```python
from build123d import *

# Parameters (mm, degrees)
SKETCH1_R           = 12.954
SKETCH1_R_2         = 2.25
SKETCH1_R_3         = 14.2748
SKETCH1_R_4         = 1.8415
BOSS_EXTRUDE1_DEPTH = 3.175
FILLET1_R           = 22.479
FILLET2_START       = -1
FILLET2_DEPTH       = 5
FILLET2_2_DEPTH     = 3.175


with BuildPart() as part:
    # Sketch1 → Boss-Extrude1 (new body)
    with BuildSketch(Plane.XY):
        Polygon((28.575, -20.461058414), (3.175, -20.461058414), (3.175, -83.961058414), (-28.575, -83.961058414), (-28.575, 55.738941586), (28.575, 55.738941586), align=None)
        with Locations((0, 33.259941586)):
            Circle(SKETCH1_R, mode=Mode.SUBTRACT)
        with Locations((0, 50.760541586)):
            Circle(SKETCH1_R_2, mode=Mode.SUBTRACT)
        with Locations((17.5006, 33.259941586)):
            Circle(SKETCH1_R_2, mode=Mode.SUBTRACT)
        with Locations((0, 15.759341586)):
            Circle(SKETCH1_R_2, mode=Mode.SUBTRACT)
        with Locations((-17.5006, 33.259941586)):
            Circle(SKETCH1_R_2, mode=Mode.SUBTRACT)
        with Locations((0, -2.935058414)):
            Circle(SKETCH1_R_3, mode=Mode.SUBTRACT)
        with Locations((-12.573, -33.351558414)):
            Circle(SKETCH1_R_4, mode=Mode.SUBTRACT)
        with Locations((-12.573, -71.451558414)):
            Circle(SKETCH1_R_4, mode=Mode.SUBTRACT)
    extrude(amount=BOSS_EXTRUDE1_DEPTH)

    # Fillet1
    fillet1_edges = [part.edges().sort_by_distance(p)[0] for p in [
        (-28.575, 55.738941586, 1.5875),
        (28.575, 55.738941586, 1.5875),
    ]]
    fillet(fillet1_edges, radius=FILLET1_R)

    # Fillet2: read off the stored shape, not the designer's step
    # Fillet2 outline → Fillet2 (cut)
    with BuildSketch(Plane.XY.offset(FILLET2_START)):
        with BuildLine():
            ThreePointArc((28.575, -7.761058414), (24.855256121, -16.741314535), (15.875, -20.461058414))
            Line((15.875, -20.461058414), (28.575, -20.461058414))
            Line((28.575, -20.461058414), (28.575, -7.761058414))
        make_face()
    extrude(amount=FILLET2_DEPTH, mode=Mode.SUBTRACT)

    # Fillet2 2 outline → Fillet2 2 (add)
    with BuildSketch(Plane.XY):
        with BuildLine():
            ThreePointArc((3.175, -33.161058414), (6.894743879, -24.180802293), (15.875, -20.461058414))
            Line((15.875, -20.461058414), (3.175, -20.461058414))
            Line((3.175, -20.461058414), (3.175, -33.161058414))
        make_face()
    extrude(amount=FILLET2_2_DEPTH)


solid = part.part
```
Design review of the part built by this model. Coordinates are the model's own, in mm. A direction names the side the tool comes from. Round coordinates to 2 decimals unless told otherwise and drop trailing zeros. Write each loop counter-clockwise with the first axis right and the second up, starting at its lowest first coordinate (ties: lowest second). Pieces come first, ordered by that corner, then holes. Notation, with made-up numbers: (-37, -13.75) -> (-32, -13.75) arc R18 cw to (-32, 6.25) -> close; hole circle Ø4 at (-26.75, 13). An arc over 180 degrees is marked (long way). Write item = value, one per line. Start each with the question number.
1) Wall thickness on probe 1 along Y at (x, z) = (0, 2.35); probe 2 along Y at (x, z) = (-5.5, 1.05); probe 3 along Y at (x, z) = (10.5, 1.6): over which ranges is each line inside the solid? List them lowest first. Write a range as from..to.
2) Take a section at D-D, the plane z = 2.6. Count the separate pieces of the cut face and the enclosed holes in it, plus the area to 3 significant figures.
3) Mouldability with a two-part tool opening along Y and no side actions: class faces 1 (the face through (22.165, 48.979, 1.61)), 2 (the face through (-12.813, -31.526, 1.565)), 3 (the face through (-28.575, -26, 2)) as +Y half, -Y half, draft (parallel to the pull), parting line (faces both ways), or undercut.
4) Tool access review of faces 4 (the face through (3.175, -58, 2)), 5 (the face through (-13, -13, 0)): name each direction out of +Z, -Z, +X, -X, +Y, -Y from which nothing blocks a thin tool from reaching the whole face with its end or side.
5) Take a section at B-B, the plane x = 11.5. State the section outline as (y, z) points (3 decimals).
6) Take a section at A-A, the plane x = 0. State the section outline as (y, z) points (3 decimals), plus the area to 3 significant figures.
7) Take a section at C-C, the plane y = 5. State the section outline as (x, z) points (3 decimals), plus the area to 3 significant figures.
Results list:
q1.probe_1 = -83.96..-17.21, 11.34..13.51, 18.01..20.31, 46.21..48.51, 53.01..55.74
q1.probe_2 = -83.96..-16.11, 10.24..21.53, 44.99..55.74
q1.probe_3 = -21.65..-12.61, 6.74..25.67, 40.85..55.3
q2.separate_pieces = 1
q2.enclosed_holes = 8
q2.area = 4,900 mm²
q3.face_1 = +Y half
q3.face_2 = undercut
q3.face_3 = draft
q4.face_4 = +Z, -Z, +X, -Y
q4.face_5 = -Z, +X, -X, +Y, -Y
q5.outline = (-21.238, 0) -> (-11.392, 0) -> (-11.392, 3.175) -> (-21.238, 3.175) -> close; (5.522, 0) -> (27.297, 0) -> (27.297, 3.175) -> (5.522, 3.175) -> close; (39.223, 0) -> (55.08, 0) -> (55.08, 3.175) -> (39.223, 3.175) -> close
q6.outline = (-83.961, 0) -> (-17.21, 0) -> (-17.21, 3.175) -> (-83.961, 3.175) -> close; (11.34, 0) -> (13.509, 0) -> (13.509, 3.175) -> (11.34, 3.175) -> close; (18.009, 0) -> (20.306, 0) -> (20.306, 3.175) -> (18.009, 3.175) -> close; (46.214, 0) -> (48.511, 0) -> (48.511, 3.175) -> (46.214, 3.175) -> close; (53.011, 0) -> (55.739, 0) -> (55.739, 3.175) -> (53.011, 3.175) -> close
q6.area = 242 mm²
q7.outline = (-28.575, 0) -> (-11.866, 0) -> (-11.866, 3.175) -> (-28.575, 3.175) -> close; (11.866, 0) -> (28.575, 0) -> (28.575, 3.175) -> (11.866, 3.175) -> close
q7.area = 106 mm²
